from build123d import *

# Parameters (mm, degrees)
F0_R     = 40
F0_R_2   = 2
F0_R_3   = 2.5
F1_DEPTH = 2


with BuildPart() as f1:
    # F0 (on Top) → F1 (new body)
    with BuildSketch(Plane.XY):
        Circle(F0_R)
        with Locations((-23, -23)):
            Circle(F0_R_2, mode=Mode.SUBTRACT)
        with Locations((23, -23)):
            Circle(F0_R_2, mode=Mode.SUBTRACT)
        with Locations((-19.5, 0)):
            Circle(F0_R_3, mode=Mode.SUBTRACT)
        with Locations((-23, 23)):
            Circle(F0_R_2, mode=Mode.SUBTRACT)
        with BuildLine():
            ThreePointArc((22, 0), (19.5, -2.5), (17, 0))
            ThreePointArc((17, 0), (19.5, 2.5), (22, 0))
        make_face(mode=Mode.SUBTRACT)
        with Locations((23, 23)):
            Circle(F0_R_2, mode=Mode.SUBTRACT)
    extrude(amount=F1_DEPTH)


solid = f1.part
Design review of the part built by this model. Coordinates are the model's own, in mm. Round coordinates to 2 decimals unless told otherwise and drop trailing zeros. Write each loop counter-clockwise with the first axis right and the second up, starting at its lowest first coordinate (ties: lowest second). Pieces come first, ordered by that corner, then holes. Notation, with made-up numbers: (-24.5, 32) -> (-1.5, 32) arc R29 ccw to (-1.5, 59) -> close; hole circle Ø10 at (3.25, 16.5). An arc over 180 degrees is marked (long way). One line per item, written item: value. Start each with the question number.
Q1. To check wall thickness, follow probe 1 along Y at (x, z) = (23, 0.6); probe 2 along Y at (x, z) = (-24, 1.3); probe 3 along Y at (x, z) = (-19.5, 1.45). State the ranges of each line that lie inside material, in increasing order.
Q2. Add section C-C (z = 1.2). Give the boundary of the cut face in (x, y).
Q3. Add section A-A (y = 0). Give the boundary of the cut face in (x, z).
Q4. Insertion check: P1, Ø4, axis at x = -19.5, y = 0, coming from the +Z side; P2, Ø1, axis at x = -24.5, z = 1, coming from the -Y side. Each pin has a flat end and moves straight along its axis. Give the tip position at first contact, or say it passes through.
Q5. Add section B-B (x = 23). Give the boundary of the cut face in (y, z).
Q6. Add section D-D (x = -19.5). Give the boundary of the cut face in (y, z).
Q7. The part is to be moulded in two halves that separate along Y. For faces 1 (the face through (-8.67, -39.05, 0.99)), 2 (the face through (-1, 1, 0)), 3 (the face through (-22, 0, 1)), say which applies: pulls with the +Y half, pulls with the -Y half, needs draft (parallel to the pull), parting line crosses it, or undercut.
Response:
1. probe 1: y = -32.73 to -25, -21 to 21, 25 to 32.73
1. probe 2: y = -32 to -24.73, -21.27 to 21.27, 24.73 to 32
1. probe 3: y = -34.92 to -2.5, 2.5 to 34.92
2. outline: circle Ø80 at (0, 0); hole circle Ø4 at (-23, -23); hole circle Ø4 at (-23, 23); hole circle Ø5 at (-19.5, 0); hole circle Ø5 at (19.5, 0); hole circle Ø4 at (23, -23); hole circle Ø4 at (23, 23)
3. outline: (-40, 0) -> (-22, 0) -> (-22, 2) -> (-40, 2) -> close; (-17, 0) -> (17, 0) -> (17, 2) -> (-17, 2) -> close; (22, 0) -> (40, 0) -> (40, 2) -> (22, 2) -> close
4. P1: passes through
4. P2: stops at y = -32
5. outline: (-32.73, 0) -> (-25, 0) -> (-25, 2) -> (-32.73, 2) -> close; (-21, 0) -> (21, 0) -> (21, 2) -> (-21, 2) -> close; (25, 0) -> (32.73, 0) -> (32.73, 2) -> (25, 2) -> close
6. outline: (-34.92, 0) -> (-2.5, 0) -> (-2.5, 2) -> (-34.92, 2) -> close; (2.5, 0) -> (34.92, 0) -> (34.92, 2) -> (2.5, 2) -> close
7. face 1: parting line crosses it
7. face 2: needs draft
7. face 3: undercut
